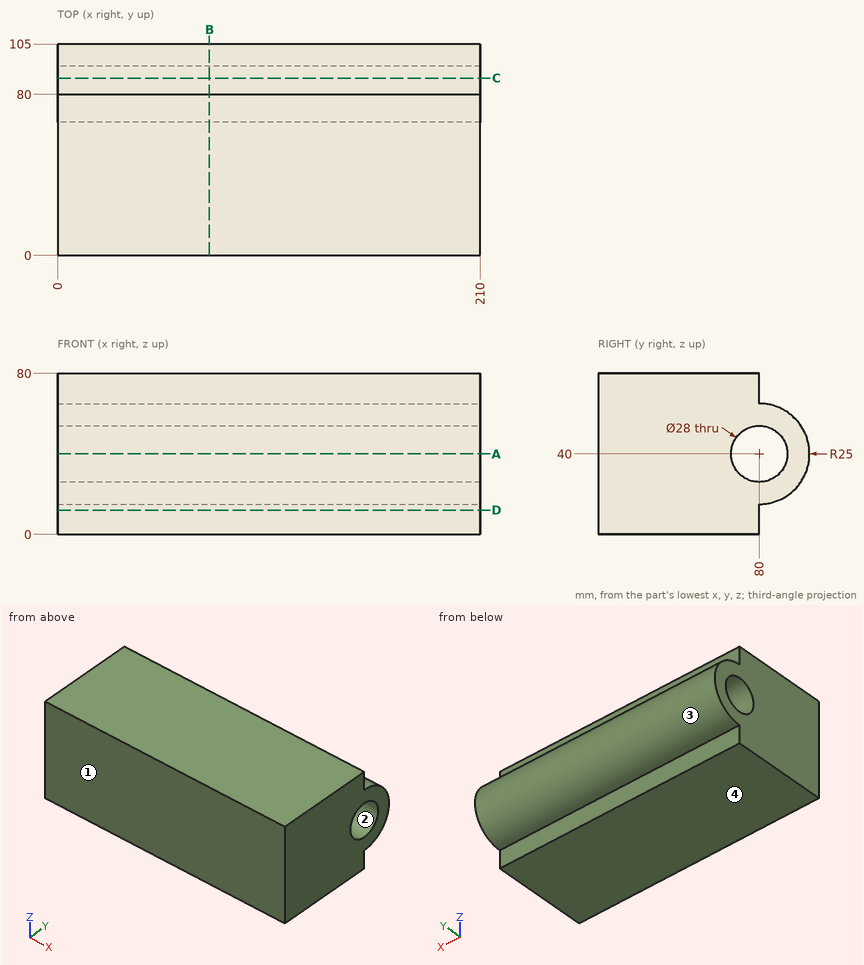
Print and shaded views of the part. All mm, measured from the part's lowest x, y and z. Round coordinates to 2 decimals unless told otherwise and drop trailing zeros. Write each loop counter-clockwise with the first axis right and the second up, starting at its lowest first coordinate (ties: lowest second). Pieces come first, ordered by that corner, then holes.
Item 1: Cut at A-A, the plane z = 40. Give the cut face in (x, y).
Results:
outline: (0, 0) - (210, 0) - (210, 66) - (0, 66) - close; (0, 94) - (210, 94) - (210, 105) - (0, 105) - close
Item 2: Two-plate mould, pull along Y, no slides. Class the marked faces 1, 2, 3 and 4: +Y half, -Y half, draft (parallel to the pull), parting line (faces both ways), or undercut.
Results:
face 1: -Y half
face 2: undercut
face 3: +Y half
face 4: draft
Item 3: Cut at B-B, the plane x = 75.5. Give the cut face in (y, z), plus the area to 3 significant figures.
Results:
outline: (0, 0) - (80, 0) - (80, 15) arc R25 ccw to (80, 65) - (80, 80) - (0, 80) - close; hole circle Ø28 at (80, 40)
area: 6,770 mm2
Item 4: Drop flat-ended pins along their axis: pin 1 Ø5 at (x, z) = (44.5, 34.5) entering from +Y; pin 2 Ø7.5 at (x, z) = (78, 6) entering from +Y. Give the stop position or say it passes through.
Results:
pin 1: stops at y = 104.82
pin 2: stops at y = 80
Item 5: Cut at D-D, the plane z = 12. Give the cut face in (x, y), plus the area to 3 significant figures.
Results:
outline: (0, 0) - (210, 0) - (210, 80) - (0, 80) - close
area: 16,800 mm2
Item 6: Probe L1, parallel to Y at x = 46, z = 40; L2, parallel to Y at x = 141, z = 38.5; L3, parallel to Z at x = 83.5, y = 81.5. List the from-to ranges inside material, lowest first.
Results:
L1: y = 0 to 66, 94 to 105
L2: y = 0 to 66.08, 93.92 to 104.95
L3: z = 15.05 to 26.08, 53.92 to 64.95
Item 7: Cut at C-C, the plane y = 88. Give the cut face in (x, z), plus the area to 3 significant figures.
Results:
outline: (0, 16.31) - (210, 16.31) - (210, 28.51) - (0, 28.51) - close; (0, 51.49) - (210, 51.49) - (210, 63.69) - (0, 63.69) - close
area: 5,120 mm2
